Can you work these out from the drawing? Everything is in mm from the part's minimum corner. A direction names the side the tool comes from. Coordinates: 2 decimals unless noted, no trailing zeros. Loops run counter-clockwise (first coordinate to the right, second up) from the corner with the lowest first, then second, coordinate; pieces in that order, holes last. Notation, with made-up numbers: (19, 8) - (54, 8) arc R12 ccw to (54, 19) - close; hole circle Ø9 at (70, 39.25). An arc over 180 degrees is marked (long way). Put each result on its own line as item: value. Start each with the question number.
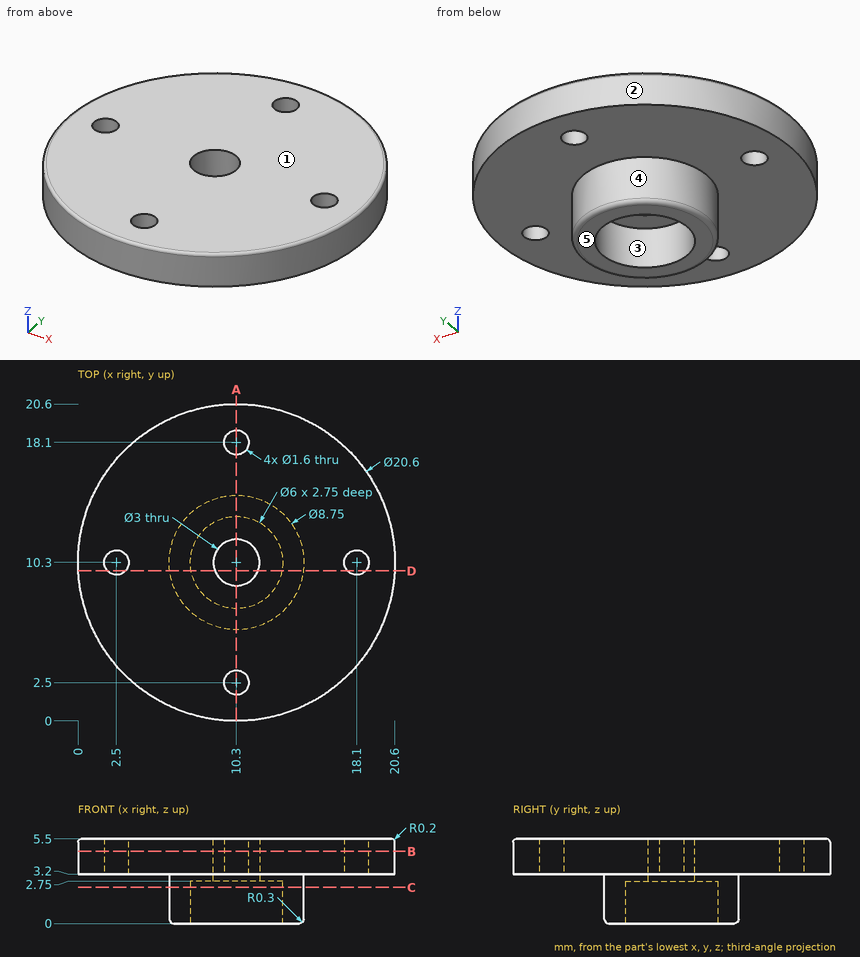
Q1. I want a section at A-A on x = 10.3. List the corners of the cut face in (y, z) for me (3 decimals).
Q2. We'd pull the mould along Y, two halves only. Please class the marked faces 1, 2 and 3: released by +Y, released by -Y, zero draft, split by the parting line, or undercut.
Q3. Please list where these lines run through material, in increasing order: line 1 along Z through (x, y) = (12.25, 14.5); line 2 along Y through (x, z) = (18.25, 4.65); line 3 along X through (y, z) = (13, 2.35). Write a range as [from, to].
Q4. Will these pins go through, and if not, where does the flat tip stop? pin 1 (1 mm diameter, centred on x = 12, y = 11, fed in from -Z); pin 2 (5 mm diameter, centred on x = 11, y = 18, fed in from -Z); pin 3 (1.3 mm diameter, centred on x = 18.1, y = 10.3, fed in from -Z); pin 4 (2 mm diameter, centred on x = 4.5, z = 3.5, fed in from +Y).
Q5. I want a section at C-C on z = 2.35. List the corners of the cut face in (x, y) for me (3 decimals), and give its area (3 significant figures).
Q6. I want a section at D-D on y = 9.75. Count the separate pieces of the cut face and the enclosed holes in it, and give its area (3 significant figures).
Q7. On a 3-axis mill with a long thin cutter (end or side, diameter ignored), from which of +Z, -Z, +X, -X, +Y, -Y can I reach the whole of each face in a straight line? I mean the marked faces 4 and 5. Say none if no direction works.
Q8. I want a section at B-B on z = 4.7. List the corners of the cut face in (x, y) for me, and give its area (3 significant figures).
Calculated:
1. outline: (0, 3.2) - (1.7, 3.2) - (1.7, 5.5) - (0.2, 5.5) arc R0.2 ccw to (0, 5.3) - close; (3.3, 3.2) - (5.925, 3.2) - (5.925, 0.3) arc R0.3 ccw to (6.225, 0) - (7.3, 0) - (7.3, 2.75) - (8.8, 2.75) - (8.8, 5.5) - (3.3, 5.5) - close; (11.8, 2.75) - (13.3, 2.75) - (13.3, 0) - (14.375, 0) arc R0.3 ccw to (14.675, 0.3) - (14.675, 3.2) - (17.3, 3.2) - (17.3, 5.5) - (11.8, 5.5) - close; (18.9, 3.2) - (20.6, 3.2) - (20.6, 5.3) arc R0.2 ccw to (20.4, 5.5) - (18.9, 5.5) - close
2. face 1: zero draft
2. face 2: split by the parting line
2. face 3: undercut
3. line 1: [3.2, 5.5]
3. line 2: [3.75, 9.51], [11.09, 16.85]
3. line 3: [6.86, 8.99], [11.61, 13.74]
4. pin 1: z = 2.75
4. pin 2: z = 3.2
4. pin 3: through
4. pin 4: y = 19.41
5. outline: circle Ø8.75 at (10.3, 10.3); hole circle Ø6 at (10.3, 10.3)
5. area: 31.9 mm2
6. separate pieces: 4
6. enclosed holes: 0
6. area: 45.8 mm2
7. face 4: -Z
7. face 5: -Z, +X, -X, +Y, -Y
8. outline: circle Ø20.6 at (10.3, 10.3); hole circle Ø1.6 at (2.5, 10.3); hole circle Ø3 at (10.3, 10.3); hole circle Ø1.6 at (10.3, 2.5); hole circle Ø1.6 at (10.3, 18.1); hole circle Ø1.6 at (18.1, 10.3)
8. area: 318 mm2
